For this review, take the finished solid that the model builds, in its own axes (mm). Coordinates: 2 decimals unless noted, no trailing zeros. Write each loop counter-clockwise with the first axis right and the second up, starting at its lowest first coordinate (ties: lowest second). Pieces come first, ordered by that corner, then holes. Notation, with made-up numbers: M -31,77 L -18,77 A17 cw -18,101 Z; hole C -26.75,11 d6. An arc over 180 degrees is marked long. One line per question, with ' | ' between items.
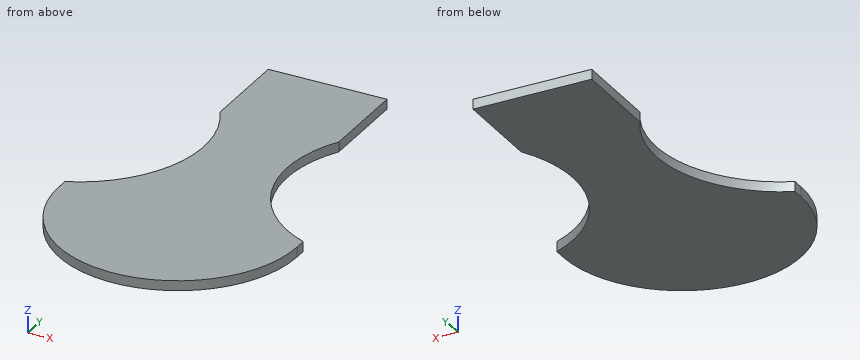
from build123d import *

# Parameters (mm, degrees)
BOSS_EXTRUDE1_DEPTH = 5
CUT_EXTRUDE1_DEPTH  = 6


with BuildPart() as part:
    # Sketch1 → Boss-Extrude1 (new body)
    with BuildSketch(Plane.XY):
        with BuildLine():
            Line((60, 65.777063513), (60, 0))
            Line((60, 0), (-60, 0))
            Line((-60, 0), (-60, 65.777063513))
            ThreePointArc((-60, 65.777063513), (-24.19023261, 103.909288798), (-29.909652169, 155.906349155))
            Line((-29.909652169, 155.906349155), (-29.909646989, 201.396349155))
            Line((-29.909646989, 201.396349155), (29.909657349, 201.396349155))
            Line((29.909657349, 201.396349155), (29.909652169, 155.906349155))
            ThreePointArc((29.909652169, 155.906349155), (24.19023261, 103.909288798), (60, 65.777063513))
        make_face()
    extrude(amount=BOSS_EXTRUDE1_DEPTH)

    # Sketch2 → Cut-Extrude1 (cut, through all)
    with BuildSketch(Plane.XY.offset(5)):
        with BuildLine():
            Line((-60, 60), (-60, -14.155296416))
            Line((-60, -14.155296416), (60, -14.155296416))
            Line((60, -14.155296416), (60, 60))
            ThreePointArc((60, 60), (0, 0), (-60, 60))
        make_face()
    extrude(amount=-CUT_EXTRUDE1_DEPTH, mode=Mode.SUBTRACT)


solid = part.part
1. Take a section at A-A on z = 3. State the section outline as (x, y) points.
Computed values:
outline: M -60,60 A60 ccw 60,60 L 60,65.78 A62.5 cw 29.91,155.91 L 29.91,201.4 L -29.91,201.4 L -29.91,155.91 A62.5 cw -60,65.78 Z
2. Take a section at B-B on y = 179.5. State the section outline as (x, z) points, plus the area to 3 significant figures.
Computed values:
outline: M -29.91,0 L 29.91,0 L 29.91,5 L -29.91,5 Z | area: 299 mm2
3. Clearance check with flat-ended pins moving along their axes: P1, Ø1.5, axis at y = 145.5, z = 1, coming from the -X side; P2, Ø1.5, axis at y = 175, z = 2.5, coming from the -X side; P3, Ø2.5, axis at y = 167.5, z = 2.5, coming from the +X side. State where each tip first meets the part, or that it passes through.
Computed values:
P1: stops at x = -25.18 | P2: stops at x = -29.91 | P3: stops at x = 29.91
4. Take a section at C-C on x = -32. State the section outline as (y, z) points, plus the area to 3 significant figures.
Computed values:
outline: M 9.25,0 L 88.25,0 L 88.25,5 L 9.25,5 Z | area: 395 mm2
5. For line 1 along X through (y, z) = (188, 1.2); line 2 along Y through (x, z) = (2, 2.75); line 3 along X through (y, z) = (41, 1.2), list the stretches that pass through material, from the lowest coordinate up.
Computed values:
line 1: x = -29.91 to 29.91 | line 2: y = 0.03 to 201.4 | line 3: x = -56.91 to 56.91
